Input: part model. Units: mm. Frame: model coordinates. A direction names the side the tool comes from. Round coordinates to 2 decimals unless told otherwise and drop trailing zeros. Write each loop counter-clockwise with the first axis right and the second up, starting at its lowest first coordinate (ties: lowest second). Pieces come first, ordered by that corner, then holes. Notation, with made-up numbers: (-21, 39) -> (13, 39) arc R6 ccw to (13, 44) -> close; hole circle Ø7 at (-38.5, -37.75). An arc over 180 degrees is marked (long way). Write item = value, one per line. Start each with the question number.
```python
from build123d import *

# Parameters (mm, degrees)
BOSS_EXTRUDE2_DEPTH     = 7
CUT_EXTRUDE2_DEPTH      = 30.130224853
CUT_EXTRUDE2_DEPTH_BACK = 30.130224853
SKETCH3_R               = 2
BOSS_EXTRUDE3_DEPTH     = 36
SKETCH5_R               = 2
BOSS_EXTRUDE4_DEPTH     = 7


with BuildPart() as part:
    # Sketch1 → Boss-Extrude2 (new body)
    with BuildSketch(Plane(origin=(0, 0, 0), x_dir=(1, 0, 0), z_dir=(0, 1, 0))):
        with BuildLine():
            Line((-24.9, 0), (-24.9, 13.4))
            Line((-24.9, 13.4), (24.9, 13.4))
            Line((24.9, 13.4), (24.9, 0))
            ThreePointArc((24.9, 0), (23.392904185, -4.800819919), (19.412411454, -7.878950407))
            Line((19.412411454, -7.878950407), (8.235013612, 1.5))
            ThreePointArc((8.235013612, 1.5), (11.116692467, 6.448255578), (16.5, 8.4))
            Line((16.5, 8.4), (-16.5, 8.4))
            ThreePointArc((-16.5, 8.4), (-11.116692467, 6.448255578), (-8.235013612, 1.5))
            Line((-8.235013612, 1.5), (-19.412411454, -7.878950407))
            ThreePointArc((-19.412411454, -7.878950407), (-23.392904185, -4.800819919), (-24.9, 0))
        make_face()
    extrude(amount=BOSS_EXTRUDE2_DEPTH)

    # Sketch3 → Cut-Extrude2 (cut, two sides: drawn at the far end of the back side and taken through both)
    with BuildSketch(Plane(origin=(0, 7, 0), x_dir=(1, 0, 0), z_dir=(0, 1, 0)).offset(-CUT_EXTRUDE2_DEPTH_BACK)):
        with Locations(Location((-16.5, 0, 0), (0, 0, 270))):
            Circle(SKETCH3_R)
        with Locations(Location((16.5, 0, 0), (0, 0, 270))):
            Circle(SKETCH3_R)
    extrude(amount=CUT_EXTRUDE2_DEPTH + CUT_EXTRUDE2_DEPTH_BACK, mode=Mode.SUBTRACT)

    # Sketch4 → Boss-Extrude3 (add)
    with BuildSketch(Plane(origin=(0, 7, 0), x_dir=(1, 0, 0), z_dir=(0, 1, 0))):
        Polygon((-24.9, 13.4), (-24.9, 0), (-20.9, 0), (-20.9, 8.4), (-16.5, 8.4), (16.5, 8.4), (20.9, 8.4), (20.9, 0), (24.9, 0), (24.9, 13.4), align=None)
    extrude(amount=BOSS_EXTRUDE3_DEPTH)

    # Sketch5 → Boss-Extrude4 (add)
    with BuildSketch(Plane(origin=(0, 43, 0), x_dir=(1, 0, 0), z_dir=(0, 1, 0))):
        with BuildLine():
            Line((-24.9, 13.4), (-24.9, 0))
            ThreePointArc((-24.9, 0), (-23.392904185, -4.800819919), (-19.412411454, -7.878950407))
            Line((-19.412411454, -7.878950407), (-8.235013612, 1.5))
            ThreePointArc((-8.235013612, 1.5), (-11.116692467, 6.448255578), (-16.5, 8.4))
            Line((-16.5, 8.4), (16.5, 8.4))
            ThreePointArc((16.5, 8.4), (11.116692467, 6.448255578), (8.235013612, 1.5))
            Line((8.235013612, 1.5), (19.412411454, -7.878950407))
            ThreePointArc((19.412411454, -7.878950407), (23.392904185, -4.800819919), (24.9, 0))
            Line((24.9, 0), (24.9, 13.4))
            Line((24.9, 13.4), (-24.9, 13.4))
        make_face()
        with Locations(Location((16.5, 0, 0), (0, 0, 270))):
            Circle(SKETCH5_R, mode=Mode.SUBTRACT)
        with Locations(Location((-16.5, 0, 0), (0, 0, 270))):
            Circle(SKETCH5_R, mode=Mode.SUBTRACT)
    extrude(amount=BOSS_EXTRUDE4_DEPTH)


solid = part.part
```
1. Pin query (flat end, axial travel): P1, Ø3, axis at x = -16.5, z = 0, coming from the +Y side; P2, Ø1.2, axis at x = 22, y = 33, coming from the +Z side; P3, Ø1.5, axis at x = -6.5, y = 28, coming from the +Z side. Return the tip coordinate at first contact, or that it passes through.
2. Section B-B (y = 45.5). Output: boundary loops of the cut face in (x, z), then the cut area to 3 significant figures.
3. Section C-C (y = 22.5). Output: boundary loops of the cut face in (x, z).
4. Line query: line 1 along Y through (x, z) = (17, -4); line 2 along Z through (x, y) = (-13, 34.5); line 3 along X through (y, z) = (43.5, 7). Output: solid intervals per line, ascending.
5. Mould query, pull axis Z, two halves, no side actions, for faces 1 (the cylindrical face through (-14.517, 46.451, -0.26)), 2 (the flat face through (24.9, 25, -7)), 3 (the cylindrical face through (-23.35, 3.45, 4.86)). Classes: pulls with the +Z half, pulls with the -Z half, needs draft (parallel to the pull), parting line crosses it, or undercut.
6. Section D-D (x = 12.5). Output: boundary loops of the cut face in (y, z), then the cut area to 3 significant figures.
7. Reachability of faces 4 (the cylindrical face through (23.434, 3.451, 4.742)), 5 (the flat face through (-16.5, 7, -2.2)), 6 (the flat face through (13.745, 46.451, 3.124)) from +Z, -Z, +X, -X, +Y, -Y: full face, straight path, thin tool, end or side. Return the list, or none.
8. Section A-A (z = 3.25). Output: boundary loops of the cut face in (x, y), then the cut area to 3 significant figures.
Check sheet entries:
q1.P1 = through
q1.P2 = 0
q1.P3 = -8.4
q2.outline = (-24.9, -13.4) -> (24.9, -13.4) -> (24.9, 0) arc R8.4 ccw to (19.41, 7.88) -> (8.24, -1.5) arc R8.4 ccw to (16.5, -8.4) -> (-16.5, -8.4) arc R8.4 ccw to (-8.24, -1.5) -> (-19.41, 7.88) arc R8.4 ccw to (-24.9, 0) -> close; hole circle Ø4 at (-16.5, 0); hole circle Ø4 at (16.5, 0)
q2.area = 610 mm2
q3.outline = (-24.9, -13.4) -> (24.9, -13.4) -> (24.9, 0) -> (20.9, 0) -> (20.9, -8.4) -> (-20.9, -8.4) -> (-20.9, 0) -> (-24.9, 0) -> close
q4.line_1 = 0 to 7, 43 to 50
q4.line_2 = -13.4 to -8.4
q4.line_3 = -21.14 to -18.36, 18.36 to 21.14
q5.face_1 = undercut
q5.face_2 = needs draft
q5.face_3 = pulls with the +Z half
q6.outline = (0, -13.4) -> (50, -13.4) -> (50, -8.4) -> (0, -8.4) -> close; (0, -7.39) -> (7, -7.39) -> (7, 2.08) -> (0, 2.08) -> close; (43, -7.39) -> (50, -7.39) -> (50, 2.08) -> (43, 2.08) -> close
q6.area = 383 mm2
q7.face_4 = +Z, +X, +Y, -Y
q7.face_5 = +Z
q7.face_6 = +Z, +Y, -Y
q8.outline = (-24.25, 0) -> (-13.9, 0) -> (-13.9, 7) -> (-24.25, 7) -> close; (-24.25, 43) -> (-13.9, 43) -> (-13.9, 50) -> (-24.25, 50) -> close; (13.9, 0) -> (24.25, 0) -> (24.25, 7) -> (13.9, 7) -> close; (13.9, 43) -> (24.25, 43) -> (24.25, 50) -> (13.9, 50) -> close
q8.area = 290 mm2
